Geometry: final body of the model. Coordinates: model frame, mm. Face numbers are marked on the shaded views. A direction names the side the tool comes from. Round coordinates to 2 decimals unless told otherwise and drop trailing zeros. Loops run counter-clockwise (first coordinate to the right, second up) from the corner with the lowest first, then second, coordinate; pieces in that order, holes last. Notation, with made-up numbers: M 56.5,34.25 L 98.5,34.25 A38 ccw 98.5,72.25 Z; hole C 62,30.5 d11. An arc over 180 degrees is marked long. Answer as a JSON object with one key per item and string values.
from build123d import *

# Parameters (mm, degrees)
SKETCH3_W           = 47.117
SKETCH3_H           = 47.117
BOSS_EXTRUDE1_DEPTH = 5.500799822
CUT_EXTRUDE2_REACH  = 7.501
SKETCH6_W           = 11
SKETCH6_H           = 11
SKETCH7_W           = 50.8
SKETCH7_H           = 50.8
SKETCH7_W_2         = 35
SKETCH7_H_2         = 35
BOSS_EXTRUDE2_DEPTH = 1.999999976
SKETCH12_W          = 35
SKETCH12_H          = 35
CUT_EXTRUDE3_DEPTH  = 3.499999912
BOSS_EXTRUDE4_DEPTH = 2.0008
FILLET3_R           = 1.5875
CUT_EXTRUDE5_DEPTH  = 5.5008


with BuildPart() as part:
    # Sketch3 → Boss-Extrude1 (new body)
    with BuildSketch(Plane(origin=(0, 0, 0), x_dir=(1, 0, 0), z_dir=(0, 1, 0))):
        with Locations((23.8125, 23.8125)):
            Rectangle(SKETCH3_W, SKETCH3_H)
    extrude(amount=BOSS_EXTRUDE1_DEPTH)

    # Sketch6 → Cut-Extrude2 (cut, up to next)
    with BuildSketch(Plane(origin=(0, 5.500799822, 0), x_dir=(1, 0, 0), z_dir=(0, 1, 0)), mode=Mode.PRIVATE) as cut_extrude2_sk1:
        with Locations((16.8125, 30.8125)):
            Rectangle(SKETCH6_W, SKETCH6_H)
    cut_extrude2_tool1 = extrude(cut_extrude2_sk1.sketch, amount=-CUT_EXTRUDE2_REACH, mode=Mode.PRIVATE) & part.part
    add(cut_extrude2_tool1.solids().sort_by_distance((16.8125, 5.5008, -30.8125))[0], mode=Mode.SUBTRACT)
    # Sketch6 → Cut-Extrude2 (cut, up to next)
    with BuildSketch(Plane(origin=(0, 5.500799822, 0), x_dir=(1, 0, 0), z_dir=(0, 1, 0)), mode=Mode.PRIVATE) as cut_extrude2_sk2:
        with Locations((30.8125, 30.8125)):
            Rectangle(SKETCH6_W, SKETCH6_H)
    cut_extrude2_tool2 = extrude(cut_extrude2_sk2.sketch, amount=-CUT_EXTRUDE2_REACH, mode=Mode.PRIVATE) & part.part
    add(cut_extrude2_tool2.solids().sort_by_distance((30.8125, 5.5008, -30.8125))[0], mode=Mode.SUBTRACT)
    # Sketch6 → Cut-Extrude2 (cut, up to next)
    with BuildSketch(Plane(origin=(0, 5.500799822, 0), x_dir=(1, 0, 0), z_dir=(0, 1, 0)), mode=Mode.PRIVATE) as cut_extrude2_sk3:
        with Locations((30.8125, 16.8125)):
            Rectangle(SKETCH6_W, SKETCH6_H)
    cut_extrude2_tool3 = extrude(cut_extrude2_sk3.sketch, amount=-CUT_EXTRUDE2_REACH, mode=Mode.PRIVATE) & part.part
    add(cut_extrude2_tool3.solids().sort_by_distance((30.8125, 5.5008, -16.8125))[0], mode=Mode.SUBTRACT)
    # Sketch6 → Cut-Extrude2 (cut, up to next)
    with BuildSketch(Plane(origin=(0, 5.500799822, 0), x_dir=(1, 0, 0), z_dir=(0, 1, 0)), mode=Mode.PRIVATE) as cut_extrude2_sk4:
        with Locations((16.8125, 16.8125)):
            Rectangle(SKETCH6_W, SKETCH6_H)
    cut_extrude2_tool4 = extrude(cut_extrude2_sk4.sketch, amount=-CUT_EXTRUDE2_REACH, mode=Mode.PRIVATE) & part.part
    add(cut_extrude2_tool4.solids().sort_by_distance((16.8125, 5.5008, -16.8125))[0], mode=Mode.SUBTRACT)

    # Sketch7 → Boss-Extrude2 (add)
    with BuildSketch(Plane(origin=(0, 5.500799822, 0), x_dir=(1, 0, 0), z_dir=(0, 1, 0))):
        with Locations((23.8125, 23.8125)):
            Rectangle(SKETCH7_W, SKETCH7_H)
        with Locations((23.8125, 23.8125)):
            Rectangle(SKETCH7_W_2, SKETCH7_H_2, mode=Mode.SUBTRACT)
    extrude(amount=BOSS_EXTRUDE2_DEPTH)

    # Sketch12 → Cut-Extrude3 (cut)
    with BuildSketch(Plane(origin=(0, 5.500799822, 0), x_dir=(1, 0, 0), z_dir=(0, 1, 0))):
        with Locations((23.8125, 23.8125)):
            Rectangle(SKETCH12_W, SKETCH12_H)
    extrude(amount=-CUT_EXTRUDE3_DEPTH, mode=Mode.SUBTRACT)

    # Sketch11 → Boss-Extrude4 (add)
    with BuildSketch(Plane(origin=(0, 2.00079991, 0), x_dir=(1, 0, 0), z_dir=(0, 1, 0))):
        Polygon((22.3125, 29.383567812), (25.3125, 29.383567812), (29.383567812, 25.3125), (29.383567812, 22.3125), (25.3125, 18.241432188), (22.3125, 18.241432188), (18.241432188, 22.3125), (18.241432188, 25.3125), align=None)
    extrude(amount=-BOSS_EXTRUDE4_DEPTH)

    # Fillet3
    fillet3_edges = [part.edges().sort_by_distance(p)[0] for p in [
        (29.383567812, 1.00039991, -22.3125),
        (25.3125, 1.00039991, -18.241432188),
        (22.3125, 1.00039991, -18.241432188),
        (18.241432188, 1.00039991, -22.3125),
        (18.241432188, 1.00039991, -25.3125),
        (22.3125, 1.00039991, -29.383567812),
        (25.3125, 1.00039991, -29.383567812),
        (29.383567812, 1.00039991, -25.3125),
        (36.3125, 1.000399955, -22.3125),
        (36.3125, 1.000399955, -11.3125),
        (25.3125, 1.000399955, -11.3125),
        (11.3125, 1.000399955, -36.3125),
        (22.3125, 1.000399955, -36.3125),
        (11.3125, 1.000399955, -25.3125),
        (22.3125, 1.000399955, -11.3125),
        (11.3125, 1.000399955, -11.3125),
        (11.3125, 1.000399955, -22.3125),
        (36.3125, 1.000399955, -25.3125),
        (25.3125, 1.000399955, -36.3125),
        (36.3125, 1.000399955, -36.3125),
        (6.3125, 4.750799854, -6.3125),
        (41.3125, 4.750799854, -6.3125),
        (41.3125, 4.750799854, -41.3125),
        (6.3125, 4.750799854, -41.3125),
        (0.254, 2.750399911, -47.371),
        (47.371, 2.750399911, -47.371),
        (47.371, 2.750399911, -0.254),
        (0.254, 2.750399911, -0.254),
    ]]
    fillet(fillet3_edges, radius=FILLET3_R)

    # Sketch13 → Cut-Extrude5 (cut)
    with BuildSketch(Plane.XZ):
        with BuildLine():
            Line((0.254, -1.8415), (0.254, -45.7835))
            ThreePointArc((0.254, -45.7835), (0.718967985, -46.906032015), (1.8415, -47.371))
            Line((1.8415, -47.371), (45.7835, -47.371))
            ThreePointArc((45.7835, -47.371), (46.906032015, -46.906032015), (47.371, -45.7835))
            Line((47.371, -45.7835), (47.371, -1.8415))
            ThreePointArc((47.371, -1.8415), (46.906032015, -0.718967985), (45.7835, -0.254))
            Line((45.7835, -0.254), (1.8415, -0.254))
            ThreePointArc((1.8415, -0.254), (0.718967985, -0.718967985), (0.254, -1.8415))
        make_face()
        with BuildLine():
            Line((4.018000092, -5.605500092), (4.018000092, -42.019499908))
            ThreePointArc((4.018000092, -42.019499908), (4.482968077, -43.142031923), (5.605500092, -43.606999908))
            Line((5.605500092, -43.606999908), (42.019499908, -43.606999908))
            ThreePointArc((42.019499908, -43.606999908), (43.142031923, -43.142031923), (43.606999908, -42.019499908))
            Line((43.606999908, -42.019499908), (43.606999908, -5.605500092))
            ThreePointArc((43.606999908, -5.605500092), (43.142031923, -4.482968077), (42.019499908, -4.018000092))
            Line((42.019499908, -4.018000092), (5.605500092, -4.018000092))
            ThreePointArc((5.605500092, -4.018000092), (4.482968077, -4.482968077), (4.018000092, -5.605500092))
        make_face(mode=Mode.SUBTRACT)
    extrude(amount=-CUT_EXTRUDE5_DEPTH, mode=Mode.SUBTRACT)


solid = part.part
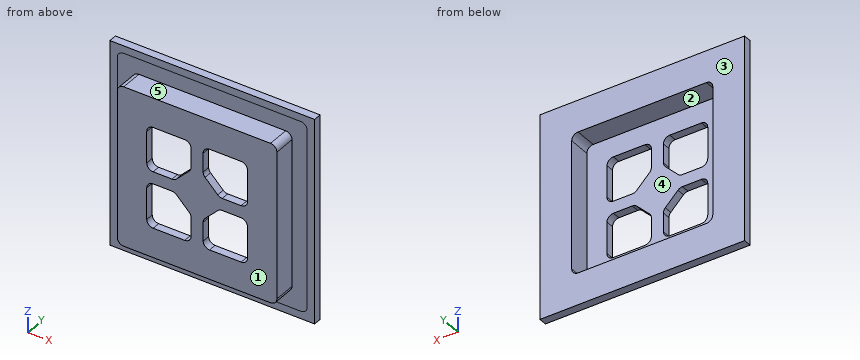
1) Ray query, line 1 (X direction, y = 6.5, z = -12.5); line 2 (Z direction, x = 32, y = 2.75); line 3 (X direction, y = 1.5, z = -27.5). Return the intervals inside material, ascending.
Results:
{"line 1": "-1.59 to 6.31, 41.31 to 49.21", "line 2": "-43.61 to -41.31, -6.31 to -4.02", "line 3": "4.02 to 11.31, 20.43 to 27.2, 36.31 to 43.61"}
2) Reachability of the marked faces 1 and 2 from +Z, -Z, +X, -X, +Y, -Y: full face, straight path, thin tool, end or side. Return the list, or none.
Results:
{"face 1": "+Z, -Z, +X, -X, -Y", "face 2": "+Y"}
3) Pin query (flat end, axial travel): P1, Ø1, axis at y = 1, z = -30, coming from the -X side; P2, Ø0.6, axis at x = 17.5, y = 0.5, coming from the -Z side; P3, Ø2, axis at x = 26.5, z = -38, coming from the +Y side. Return the tip coordinate at first contact, or that it passes through.
Results:
{"P1": "x = 4.02", "P2": "z = -43.61", "P3": "y = 2"}
4) Pull-direction query (Z, two-part tool) for the marked faces 3, 4 and 5; classes: +Z half, -Z half, draft (parallel to the pull), parting line (faces both ways), or undercut.
Results:
{"face 3": "draft", "face 4": "undercut", "face 5": "+Z half"}
5) Section query D-D (x = 38). Return the cut outline in (y, z), and give its area (3 significant figures).
Results:
{"outline": "M 0,-43.61 L 5.5,-43.61 L 5.5,-49.21 L 7.5,-49.21 L 7.5,-41.31 L 2,-41.31 L 2,-6.31 L 7.5,-6.31 L 7.5,1.59 L 5.5,1.59 L 5.5,-4.02 L 0,-4.02 Z", "area": "127 mm2"}
6) Section query B-B (z = -15.5). Return the cut outline in (x, y), and give its area (3 significant figures).
Results:
{"outline": "M -1.59,5.5 L 4.02,5.5 L 4.02,0 L 11.31,0 L 11.31,2 L 6.31,2 L 6.31,7.5 L -1.59,7.5 Z; M 22.31,0 L 25.31,0 L 25.31,2 L 22.31,2 Z; M 36.31,0 L 43.61,0 L 43.61,5.5 L 49.21,5.5 L 49.21,7.5 L 41.31,7.5 L 41.31,2 L 36.31,2 Z", "area": "82.9 mm2"}
7) Section query A-A (y = 4.5). Return the cut outline in (x, z) (1 decimal), and give its area (3 significant figures).
Results:
{"outline": "M 4,-42 A1.6 ccw 5.6,-43.6 L 42,-43.6 A1.6 ccw 43.6,-42 L 43.6,-5.6 A1.6 ccw 42,-4 L 5.6,-4 A1.6 ccw 4,-5.6 Z; hole M 6.3,-39.7 A1.6 ccw 7.9,-41.3 L 39.7,-41.3 A1.6 ccw 41.3,-39.7 L 41.3,-7.9 A1.6 ccw 39.7,-6.3 L 7.9,-6.3 A1.6 ccw 6.3,-7.9 Z", "area": "342 mm2"}
8) Section query C-C (x = 13.5). Return the cut outline in (y, z).
Results:
{"outline": "M 0,-43.61 L 5.5,-43.61 L 5.5,-49.21 L 7.5,-49.21 L 7.5,-41.31 L 2,-41.31 L 2,-36.31 L 0,-36.31 Z; M 0,-25.31 L 2,-25.31 L 2,-22.31 L 0,-22.31 Z; M 0,-11.31 L 2,-11.31 L 2,-6.31 L 7.5,-6.31 L 7.5,1.59 L 5.5,1.59 L 5.5,-4.02 L 0,-4.02 Z"}
